Can you work these out from the model? Positions are in its coordinate system, mm. A direction names the side the tool comes from. Round coordinates to 2 decimals unless told otherwise and drop trailing zeros. Order: outer loops, then holes, each group sorted by start corner. A loop starts at its lowest first (then second) coordinate and runs counter-clockwise, first axis right, second up.
Q1. If we section it at D-D (z = -3.95): Please give me the cut outline in (x, y).
Q2. If we section it at C-C (y = -1.75): Please give me the cut outline in (x, z).
Q3. If I drill on line 1 (X direction, y = -1.75, z = -3.55); line 2 (Y direction, x = 6.75, z = -3.85); line 3 (X direction, y = 1.75, z = -2.55), over which ranges is the centre line in solid material (lowest first)?
Q4. For faces 1 (the face through (6, 3, -2)), 2 (the face through (4, 3, -2)), 3 (the face through (5, 3, -3.25)), 4 (the face through (3.25, -2, -2)), 5 (the face through (12, 0, -2)), which set-ups out of +Z, -Z, +X, -X, +Y, -Y let a thin tool reach every point of the face, with its end or its side?
Q5. Will these pins go through, and if not, where does the flat tip stop? P1, Ø1, axis at y = 2, z = -2.5, coming from the +X side; P2, Ø1.6, axis at x = 5.5, y = 3, coming from the -Z side; P3, Ø2.5, axis at x = 12.5, z = -2.5, coming from the -Y side.
Q6. If we section it at B-B (x = 4.5): Please give me the cut outline in (y, z), plus the area to 3 significant figures.
Q7. If we section it at A-A (z = -2.15): Please give me the cut outline in (x, y), plus the area to 3 significant figures.
from build123d import *

# Parameters (mm, degrees)
CROQUIS1_W              = 14
CROQUIS1_H              = 4.5
SALIENTE_EXTRUIR1_DEPTH = 1
CROQUIS2_W              = 7.5
CROQUIS2_H              = 4.5
SALIENTE_EXTRUIR2_DEPTH = 6
CROQUIS3_W              = 2
CROQUIS3_H              = 2
SALIENTE_EXTRUIR3_DEPTH = 4


with BuildPart() as part:
    # Croquis1 → Saliente-Extruir1 (new body)
    with BuildSketch(Plane(origin=(0, 0, 0), x_dir=(1, 0, 0), z_dir=(0, 1, 0))):
        with Locations((7, 2.25)):
            Rectangle(CROQUIS1_W, CROQUIS1_H)
    extrude(amount=SALIENTE_EXTRUIR1_DEPTH)

    # Croquis2 → Saliente-Extruir2 (add)
    with BuildSketch(Plane(origin=(0, 1, 0), x_dir=(1, 0, 0), z_dir=(0, 1, 0))):
        with Locations((7, 2.25)):
            Rectangle(CROQUIS2_W, CROQUIS2_H)
    extrude(amount=-SALIENTE_EXTRUIR2_DEPTH)

    # Croquis3 → Saliente-Extruir3 (add)
    with BuildSketch(Plane(origin=(0, 1, 0), x_dir=(1, 0, 0), z_dir=(0, 1, 0))):
        with Locations((5, 2.25)):
            Rectangle(CROQUIS3_W, CROQUIS3_H)
    extrude(amount=SALIENTE_EXTRUIR3_DEPTH)


solid = part.part
Solution:
1. outline: (0, 0) - (3.25, 0) - (3.25, -5) - (10.75, -5) - (10.75, 0) - (14, 0) - (14, 1) - (0, 1) - close
2. outline: (3.25, -4.5) - (10.75, -4.5) - (10.75, 0) - (3.25, 0) - close
3. line 1: x = 3.25 to 10.75
3. line 2: y = -5 to 1
3. line 3: x = 4 to 6
4. face 1: +Z, -Z, +X, +Y
4. face 2: +Z, -Z, -X, +Y
4. face 3: -Z, +X, -X, +Y
4. face 4: +Z, -Z, -X, -Y
4. face 5: +Z, -Z, +X, -Y
5. P1: stops at x = 6
5. P2: stops at z = -3.25
5. P3: stops at y = 0
6. outline: (-5, -4.5) - (1, -4.5) - (1, -3.25) - (5, -3.25) - (5, -1.25) - (1, -1.25) - (1, 0) - (-5, 0) - close
6. area: 35.0 mm2
7. outline: (0, 0) - (3.25, 0) - (3.25, -5) - (10.75, -5) - (10.75, 0) - (14, 0) - (14, 1) - (6, 1) - (6, 5) - (4, 5) - (4, 1) - (0, 1) - close
7. area: 59.5 mm2
